```python
from build123d import *

# Parameters (mm, degrees)
ZAOKR_GLENIE1_R            = 6
OTW_R_GWINTOWANY_M51_D     = 4.2
OTW_R_GWINTOWANY_M51_DEPTH = 14
OTW_R_GWINTOWANY_M51_TIP   = 1.2618073


with BuildPart() as part:
    # Szkic1 → Obrót1 (revolve)
    with BuildSketch(Plane.XY):
        with BuildLine():
            Line((0, 0), (12.5, 0))
            Line((12.5, 0), (12.5, 8))
            ThreePointArc((12.5, 8), (9.671572875, 9.171572875), (8.5, 12))
            Line((8.5, 12), (8.5, 13.89613301))
            ThreePointArc((8.5, 13.89613301), (8.958043684, 15.754773764), (10.227272727, 17.18774519))
            ThreePointArc((10.227272727, 17.18774519), (17.18459465, 37.356277318), (0, 50))
            Line((0, 50), (0, 0))
        make_face()
    revolve(axis=Axis((0, 0, 0), (0, 1, 0)))

    # Zaokrąglenie1
    zaokr_glenie1_edges = [part.edges().sort_by_distance(p)[0] for p in [
        (-12.5, 8, 0),
    ]]
    fillet(zaokr_glenie1_edges, radius=ZAOKR_GLENIE1_R)

    # Otwór gwintowany M51
    with Locations(Plane(origin=(0, 0, 0), x_dir=(-1, 0, 0), z_dir=(0, -1, 0))):
        with Locations((0, 0)):
            Hole(OTW_R_GWINTOWANY_M51_D / 2, depth=OTW_R_GWINTOWANY_M51_DEPTH)
            with Locations((0, 0, -(OTW_R_GWINTOWANY_M51_DEPTH + OTW_R_GWINTOWANY_M51_TIP / 2))):  # 118° drill point
                Cone(0, OTW_R_GWINTOWANY_M51_D / 2, OTW_R_GWINTOWANY_M51_TIP, mode=Mode.SUBTRACT)


solid = part.part
```
Part model, mm, in its own coordinate system. A direction names the side the tool comes from. Round coordinates to 2 decimals unless told otherwise and drop trailing zeros. Loops run counter-clockwise (first coordinate to the right, second up) from the corner with the lowest first, then second, coordinate; pieces in that order, holes last. Notation, with made-up numbers: (65, 35.25) -> (106, 35.25) arc R32 ccw to (106, 68.25) -> close; hole circle Ø4 at (22, -21.75). An arc over 180 degrees is marked (long way). Use one line per item in the form item = value. Start each with the question number.
Item 1: Band-saw the part on B-B (y = 19). List the corners of the cut face in (x, z).
Item 2: Drop flat-ended pins along their axis: pin 1 Ø6 at (x, z) = (-1.5, 14) entering from +Y; pin 2 Ø8 at (x, y) = (8, 27.5) entering from +Z; pin 3 Ø1.5 at (x, y) = (-7, 9) entering from +Z. Give the stop position or say it passes through.
Item 3: Two-plate mould, pull along Y, no slides. Class faces 1 (the cylindrical face through (2.003, 7.098, -0.631)), 2 (the cylindrical face through (4.57, 12.961, -7.167)), 3 (the conical face through (-0.34, 15.04, 0.14)): released by +Y, released by -Y, zero draft, split by the parting line, or undercut.
Item 4: Band-saw the part on A-A (x = 14). List the corners of the cut face in (y, z).
Item 5: Tool access for faces 4 (the cylindrical face through (11.923, 2.028, -3.755)), 5 (the flat face through (0, 0, 3)): list every direction of +Z, -Z, +X, -X, +Y, -Y with a clear straight run to the whole face (end or side of a thin tool).
Item 6: Drill centre lines: line 1 along Z through (x, y) = (0, 8.5); line 2 along Y through (x, z) = (8.5, -2.5); line 3 along Y through (x, z) = (-7, -8.5). Where is each one in solid material? Low to high.
Data:
q1.outline = circle Ø24.9 at (0, 0)
q2.pin_1 = 46.19
q2.pin_2 = 17.24
q2.pin_3 = 8.32
q3.face_1 = zero draft
q3.face_2 = undercut
q3.face_3 = released by -Y
q4.outline = circle Ø22.63 at (32, 0)
q5.face_4 = -Y
q5.face_5 = +Z, -Z, +X, -X, -Y
q6.line_1 = -10.47 to -2.1, 2.1 to 10.47
q6.line_2 = 0 to 10.34, 15.55 to 47.67
q6.line_3 = 0 to 7.96, 17.76 to 46.24
